CAD build for the part. Positions are in the model's coordinates, mm. A direction names the side the tool comes from. Coordinates: 2 decimals unless noted, no trailing zeros. Order: outer loops, then holes, each group sorted by start corner. A loop starts at its lowest first (then second) coordinate and runs counter-clockwise, first axis right, second up. Notation, with made-up numbers: M -31.5,15 L -8.5,15 A28 cw -8.5,41 Z; hole C 82,68.25 d10. An arc over 180 degrees is marked long. One line per item, written item: value.
from build123d import *

# Parameters (mm, degrees)
F0_W     = 88.9
F0_H     = 31.8
F0_R     = 2.125
F1_DEPTH = 6.4
F2_W     = 88.9
F2_H     = 38.2
F2_R     = 2.125
F3_DEPTH = 6.4
F4_SIZE  = 1.5


with BuildPart() as f1:
    # F0 (on Top) → F1 (new body)
    with BuildSketch(Plane.XY):
        Rectangle(F0_W, F0_H)
        with Locations((-28.45, 6.5)):
            Circle(F0_R, mode=Mode.SUBTRACT)
        with Locations((0, 6.5)):
            Circle(F0_R, mode=Mode.SUBTRACT)
        with Locations((28.45, 6.5)):
            Circle(F0_R, mode=Mode.SUBTRACT)
    extrude(amount=F1_DEPTH)

    # F2 (on face) → F3 (join)
    with BuildSketch(Plane.XZ.offset(15.9)):
        with Locations((0, 19.1)):
            Rectangle(F2_W, F2_H)
        with Locations((-28.45, 22.4)):
            Circle(F2_R, mode=Mode.SUBTRACT)
        with Locations((0, 22.4)):
            Circle(F2_R, mode=Mode.SUBTRACT)
        with Locations((28.45, 22.4)):
            Circle(F2_R, mode=Mode.SUBTRACT)
    extrude(amount=F3_DEPTH)

    # F4
    f4_edges = [f1.edges().sort_by_distance(p)[0] for p in [
        (0, -22.3, 38.2),
        (0, -22.3, 0),
        (0, 15.9, 0),
        (44.45, -3.2, 0),
        (44.45, 15.9, 3.2),
        (-44.45, 15.9, 3.2),
        (-44.45, -3.2, 0),
        (-44.45, -22.3, 19.1),
        (44.45, -22.3, 19.1),
        (-44.45, -19.1, 38.2),
        (44.45, -19.1, 38.2),
    ]]
    chamfer(f4_edges, length=F4_SIZE)


solid = f1.part
Q1. Slice it at B-B (y = 6.5). List the corners of the cut face in (x, z) (3 decimals).
Recorded:
outline: M -44.45,1.5 L -42.95,0 L -30.575,0 L -30.575,6.4 L -44.45,6.4 Z; M -26.325,0 L -2.125,0 L -2.125,6.4 L -26.325,6.4 Z; M 2.125,0 L 26.325,0 L 26.325,6.4 L 2.125,6.4 Z; M 30.575,0 L 42.95,0 L 44.45,1.5 L 44.45,6.4 L 30.575,6.4 Z
Q2. Drill centre lines: line 1 along X through (y, z) = (6, 3); line 2 along X through (y, z) = (-20.5, 21); line 3 along Y through (x, z) = (0, 2.5) (3 decimals). Where is each one in solid material? Low to high.
Recorded:
line 1: x = -44.45 to -30.52, -26.38 to -2.07, 2.07 to 26.38, 30.52 to 44.45
line 2: x = -44.45 to -30.05, -26.85 to -1.6, 1.6 to 26.85, 30.05 to 44.45
line 3: y = -22.3 to 4.375, 8.625 to 15.9
Q3. Slice it at C-C (x = -28.45). List the corners of the cut face in (y, z) (3 decimals), plus the area to 3 significant figures.
Recorded:
outline: M -22.3,1.5 L -20.8,0 L 4.375,0 L 4.375,6.4 L -15.9,6.4 L -15.9,20.275 L -22.3,20.275 Z; M -22.3,24.525 L -15.9,24.525 L -15.9,38.2 L -20.8,38.2 L -22.3,36.7 Z; M 8.625,0 L 14.4,0 L 15.9,1.5 L 15.9,6.4 L 8.625,6.4 Z
area: 390 mm^2
Q4. Mould opens along Y. For faces 3 (the face through (-44.45, -10, 6)), 4 (the face through (-0.461, 4.426, 3.155)), 5 (the face through (29.4, 4.6, 3.2)), 6 (the face through (-1, -22.3, 19)) say: released by +Y, released by -Y, zero draft, split by the parting line, or undercut.
Recorded:
face 3: zero draft
face 4: undercut
face 5: undercut
face 6: released by -Y
Q5. Which spindle directions (+Z, -Z, +X, -X, +Y, -Y) get a long thin tool onto all of the face, cutting with end or side? Do faces 1 (the face through (-1, -3, 0)), 2 (the face through (-1, 0, 6.4)). Say none if no direction does.
Recorded:
face 1: -Z, +X, -X, +Y, -Y
face 2: +Z, +X, -X, +Y
Q6. Pin check, flat tips, straight feed: pin 1 Ø1.5 at (x, z) = (7.5, 19.5) entering from +Y; pin 2 Ø3 at (x, y) = (-3.5, -4.5) entering from +Z. Stop position of each tip, or through.
Recorded:
pin 1: stops at y = -15.9
pin 2: stops at z = 6.4
Q7. Slice it at D-D (z = 29). List the corners of the cut face in (x, y), plus the area to 3 significant figures.
Recorded:
outline: M -44.45,-20.8 L -42.95,-22.3 L 42.95,-22.3 L 44.45,-20.8 L 44.45,-15.9 L -44.45,-15.9 Z
area: 567 mm^2
Q8. Slice it at A-A (z = 22.4). List the corners of the cut face in (x, y) (3 decimals), plus the area to 3 significant figures.
Recorded:
outline: M -44.45,-20.8 L -42.95,-22.3 L -30.575,-22.3 L -30.575,-15.9 L -44.45,-15.9 Z; M -26.325,-22.3 L -2.125,-22.3 L -2.125,-15.9 L -26.325,-15.9 Z; M 2.125,-22.3 L 26.325,-22.3 L 26.325,-15.9 L 2.125,-15.9 Z; M 30.575,-22.3 L 42.95,-22.3 L 44.45,-20.8 L 44.45,-15.9 L 30.575,-15.9 Z
area: 485 mm^2
